Geometry: final body of the model. Coordinates: model frame, mm. Face numbers are marked on the shaded views. A direction names the side the tool comes from. Give positions to 0.01 mm unless a question says otherwise; leave off trailing zeros. Write each loop counter-clockwise with the first axis right and the second up, starting at its lowest first coordinate (ties: lowest second). Pieces come first, ordered by that corner, then holes. Notation, with made-up numbers: M 14,-29 L 37,-29 A23 cw 37,-5 Z; hole C 46,36 d10. An arc over 180 degrees is marked long. One line per question, with ' | ' between items.
Autodesk Inventor part; units mm, degrees
ref_plane "YZ Plane" through (0, 0, 0) normal (1, 0, 0) x (0, 1, 0)
ref_plane "XZ Plane" through (0, 0, 0) normal (0, 1, 0) x (-1, 0, 0)
ref_plane "XY Plane" through (0, 0, 0) normal (0, 0, 1) x (1, 0, 0)
sketch "Sketch1" plane through (0, 0, 0) normal (1, 0, 0) x (0, 1, 0)
  line L0 (-22.6931, 110) -> (55.0359, 110)
  line L1 (55, -110) -> (-22.6931, -110)
  line L2 (-62.7298, 0) -> (-22.6931, -110)
  line L3 (-62.7298, 0) -> (-22.6931, 110)
  line L4 (-57.4089, 0) -> (-19.449, -104.2938)
  line L5 (-14.4482, -105) -> (55, -105)
  line L6 (55.0359, 105) -> (-14.4122, 105)
  line L7 (-19.449, 104.2938) -> (-57.4089, 0)
  line L8 (55.0034, 17.6855) -> (-14.4593, 17.6855)
  line L9 (55.0034, 22.5) -> (-14.4456, 22.5496)
  line L10 (55, -52.5) -> (-14.449, -52.5)
  line L11 (55, -47.6855) -> (-14.449, -47.7352)
  line L12 (-60.6224, -5.7899) -> (-60, -7.5)
  line L13 (-60.6224, 5.7899) -> (-60, 7.5)
  line L14 (-14.4122, 105) -> (-14.4122, 68.1255)
  line L15 (-14.4456, 59.4672) -> (-14.4456, 22.5496)
  line L16 (-19.449, 104.2938) -> (-19.449, 68.1255)
  line L17 (-14.4593, 17.6855) -> (-14.4593, -10.5317)
  line L18 (-14.449, -19.4683) -> (-14.449, -47.7352)
  line L19 (-19.4705, 59.4672) -> (-19.4705, -10.5317)
  line L20 (-14.449, -52.5) -> (-14.449, -74.4672)
  line L21 (-14.4482, -83.1255) -> (-14.4482, -105.0928)
  line L22 (-19.4499, -19.4683) -> (-19.4499, -74.4672)
  line L23 (-19.449, -83.1255) -> (-19.449, -104.2938)
  line L24 (-19.449, -74.4672) -> (-19.4499, -74.4672)
  line L25 (-14.4593, -83.1255) -> (-14.4482, -83.1255)
  line L26 (-19.4499, -19.4683) -> (-19.449, -19.4683)
  line L27 (-19.4705, -10.5317) -> (-19.449, -10.5317)
  line L28 (-14.4122, 68.1255) -> (-14.4125, 68.1255)
  line L29 (-19.4705, 59.4672) -> (-19.449, 59.4672)
  line L30 (55.0359, 105) -> (55.0359, 110)
  line L31 (55.0034, 22.5) -> (55.0034, 17.6855)
  line L32 (55, -47.6855) -> (55, -52.5)
  line L33 (55, -105) -> (55, -110)
  line L34 (-19.449, -91.3967) -> (-19.449, 76.5553)
  line L35 (-14.4122, 69.213) -> (-14.4225, 22.5496)
  line L36 (-14.4236, 17.6855) -> (-14.438, -47.7351)
  line L37 (-14.439, -52.5) -> (-14.4482, -94.1091)
  point P0 (0, 0)
extrude "Extrusion1" add sketch "Sketch1" along normal blind 170
sketch "Sketch2" plane through (0, -14.4236, 17.6855) normal (0, 1, -0.0002) x (1, 0, 0)
  circle A0 centre (80, 33.4744) radius 10
  circle A1 centre (80, 98.5003) radius 10
  circle A2 centre (80, -44.9284) radius 10
  point P0 (0, 17.6824)
  dimension "d24" = 20
  dimension "d25" = 20
  dimension "d26" = 20
extrude "Extrusion2" cut sketch "Sketch2" against normal blind 6
sketch "Sketch3" plane through (0, -22.6931, -110) normal (0, -0.9397, -0.342) x (1, 0, 0)
  point P0 (0, 95.6047)
sketch "Sketch4" plane through (0, -22.6931, -110) normal (0, -0.9397, -0.342) x (1, 0, 0)
  line L0 (0, 117.1568) -> (170, 117.1568)
  circle A0 centre (85, 117.1568) radius 7.5
  point P0 (0, 95.6047)
  dimension "d29" = 15
extrude "Extrusion3" cut sketch "Sketch4" against normal blind 10
sketch "Sketch5" plane through (0, 0, 0) normal (-1, 0, 0) x (0, 0, 1)
  line L0 (-110, -22.6931) -> (-110, 55)
  line L1 (-110, 55) -> (109.7253, 55)
  line L2 (109.7253, 55) -> (109.7253, -62.9244)
  line L3 (109.7253, -62.9244) -> (-110, -62.9244)
  line L4 (-110, -62.9244) -> (-110, 55)
  point P0 (0, 0)
extrude "Extrusion4" add sketch "Sketch5" along normal blind 5
sketch "Sketch6" plane through (170, 0, 0) normal (1, 0, 0) x (0, 0, -1)
  line L0 (-109.7253, 55) -> (-109.7253, -22.793)
  line L1 (110, -22.6931) -> (110, -62.9244)
  line L2 (-109.7253, 55) -> (110, 55)
  line L3 (110, 55) -> (110, -62.9244)
  line L4 (110, -62.9244) -> (-109.7253, -62.9244)
  line L5 (-109.7253, -62.9244) -> (-109.7253, 55)
  point P0 (0, 0)
extrude "Extrusion5" add sketch "Sketch6" along normal blind 5
sketch "Sketch7" plane through (0, -62.9244, 109.7253) normal (0, 0, 1) x (1, 0, 0)
  line L0 (-5, 117.9244) -> (175, 117.9244)
  line L1 (-5, 117.9244) -> (175, 117.9244)
  line L2 (175, 117.9244) -> (175, 0)
  line L3 (175, 0) -> (-5, 0)
  line L4 (-5, 0) -> (-5, 117.9244)
  line L5 (175, 0) -> (-5, 0)
  line L6 (-5, 0) -> (-5, 117.9244)
  line L7 (-5, 117.9244) -> (175, 117.9244)
  line L8 (175, 117.9244) -> (175, 0)
  point P0 (0, 62.9244)
sketch "Sketch8" plane through (0, -22.6931, 110) normal (0, -0.9397, 0.342) x (1, 0, 0)
  circle A0 centre (144.5406, -21.5508) radius 6.0469
  point P0 (0, -95.6047)
extrude "Extrusion6" cut sketch "Sketch8" against normal blind 6
sketch "Sketch9" plane through (0, -62.9244, -110) normal (0, 0, -1) x (-1, 0, 0)
  line L0 (-175, 117.9244) -> (-175, 0)
  line L1 (0, 117.9244) -> (5, 117.9244)
  line L2 (-175, 0) -> (5, 0)
  line L3 (5, 0) -> (5, 117.9244)
  line L4 (5, 117.9244) -> (-175, 117.9244)
  line L5 (-175, 117.9244) -> (-175, 0)
  point P0 (0, 62.9244)
  point P1 (-175, 117.9244)
extrude "Extrusion7" add sketch "Sketch9" along normal blind 5
properties part number "container unit" material "Pine, Southern"
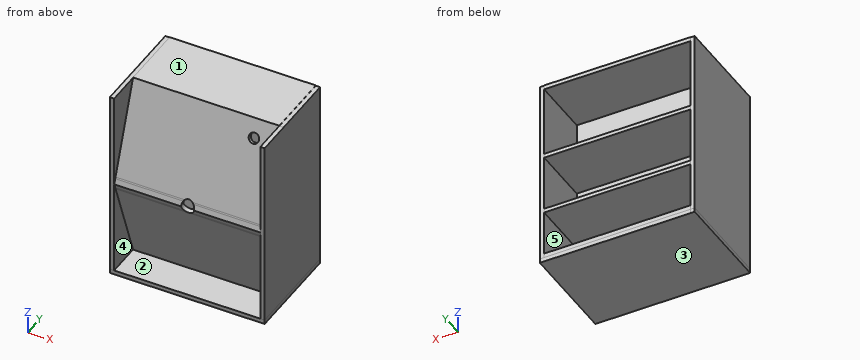
(1) Material intervals for L1, parallel to Z at x = 80, y = -17; L2, parallel to Z at x = 137.5, y = -7; L3, parallel to X at y = -27, z = -53, sorted ascending. Write a range as [from, to].
Working result:
L1: z = [-115, -90.81], [-70.81, -25.79], [-5.79, 52.61], [72.61, 110] | L2: z = [-115, -105], [-52.5, -47.73], [17.69, 22.54], [105, 110] | L3: x = [-5, 0], [170, 175]
(2) Cut plane C-C, the plane y = -7. Return loops of the section in (x, z), then the cut area to 3 significant figures.
Working result:
outline: M -5,-115 L 175,-115 L 175,109.73 L 170,109.73 L 170,110 L 0,110 L 0,109.73 L -5,109.73 Z; hole M 0,-105 L 170,-105 L 170,-52.5 L 0,-52.5 Z; hole M 0,-47.73 L 170,-47.73 L 170,17.69 L 0,17.69 Z; hole M 0,22.54 L 170,22.54 L 170,105 L 0,105 Z | area: 6,430 mm^2
(3) First-contact query: P1, Ø12, axis at x = 17.5, z = 29, coming from the +Y side; P2, Ø12, axis at x = 80, z = -15.79, coming from the +Y side; P3, Ø9.5, axis at x = 144.5, z = 62, coming from the -Y side; P4, Ø5.5, axis at x = -1.5, y = 6.5, coming from the +Z side. Flat tips, straight axial feed; report the tip coordinate or a pass-through.
Working result:
P1: stops at y = -14.42 | P2: stops at y = -49.48 | P3: stops at y = -41.89 | P4: stops at z = 110
(4) Cut plane A-A, the plane y = -45. Return loops of the section in (x, z), then the cut area to 3 significant figures.
Working result:
outline: M -5,-115 L 175,-115 L 175,109.73 L 170,109.73 L 170,48.71 L 0,48.71 L 0,109.73 L -5,109.73 Z; hole M 0,-110 L 170,-110 L 170,-48.71 L 0,-48.71 Z; hole M 0,-34.09 L 170,-34.09 L 170,34.09 L 0,34.09 Z | area: 8,070 mm^2
(5) Draft query along Z for the marked faces 1, 2 and 3. Return one class per face: released by +Z, released by -Z, zero draft, split by the parting line, or undercut.
Working result:
face 1: released by +Z | face 2: undercut | face 3: released by -Z
(6) Set-up query: the marked faces 4 and 5. Return all of +Z, -Z, +X, -X, +Y, -Y with unobstructed straight access to the full face (end or side cutting, diameter ignored); none if empty.
Working result:
face 4: -Y | face 5: +Y
